Model file for the job. Use its own axes, mm. Coordinates: 2 decimals unless noted, no trailing zeros. Loops run counter-clockwise (first coordinate to the right, second up) from the corner with the lowest first, then second, coordinate; pieces in that order, holes last. Notation, with made-up numbers: (13.5, 22.25) -> (39.5, 22.25) arc R19 ccw to (39.5, 41.25) -> close; hole circle Ø11 at (40.5, -4.75). An arc over 180 degrees is marked (long way). Use one line per item in the form item = value.
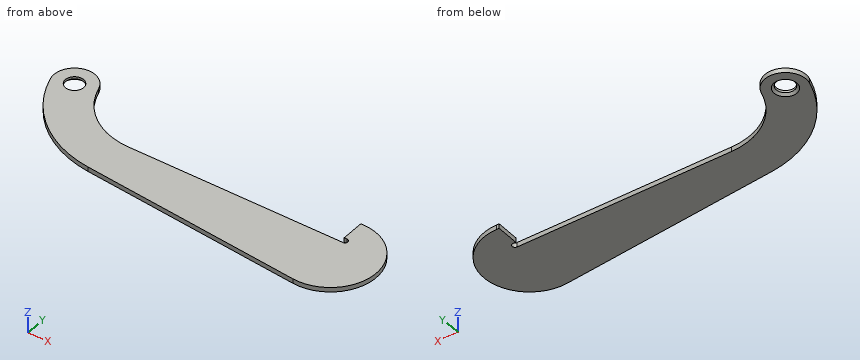
```python
from build123d import *

# Parameters (mm, degrees)
SKETCH_1_R             = 8
SM_BASE_FLANGE_1_DEPTH = 4
CHAMFER_2_SIZE         = 2


# Sheet-metal steps are written as plain solids
with BuildPart() as part:
    # Sketch 1 → Базовая кромка1 (new body)
    with BuildSketch(Plane.XY):
        with BuildLine():
            Line((259.153254995, -11.814954576), (261.653254995, -11.814954576))
            ThreePointArc((261.653254995, -11.814954576), (301.603884083, -53.801719646), (257.684629276, -91.617592804))
            Line((257.684629276, -91.617592804), (64.398882219, -72.345533941))
            ThreePointArc((64.398882219, -72.345533941), (13.404361157, -51.155129463), (-17.229741187, -5.209224379))
            ThreePointArc((-17.229741187, -5.209224379), (-5.209224379, 17.229741187), (17.229741187, 5.209224379))
            ThreePointArc((17.229741187, 5.209224379), (38.587121714, -25.160558799), (73.838171235, -36.814954576))
            Line((73.838171235, -36.814954576), (261.653254995, -36.814954576))
            ThreePointArc((261.653254995, -36.814954576), (264.153254995, -34.314954576), (261.653254995, -31.814954576))
            Line((261.653254995, -31.814954576), (259.153254995, -31.814954576))
            Line((259.153254995, -31.814954576), (259.153254995, -11.814954576))
        make_face()
        Circle(SKETCH_1_R, mode=Mode.SUBTRACT)
    extrude(amount=SM_BASE_FLANGE_1_DEPTH)

    # Фаска2
    chamfer_2_edges = [part.edges().sort_by_distance(p)[0] for p in [
        (-8, 0, 0),
    ]]
    chamfer(chamfer_2_edges, length=CHAMFER_2_SIZE)


solid = part.part
```
Q1. Pin check, flat tips, straight feed: pin 1 Ø0.8 at (x, z) = (261, 2.5) entering from +Y; pin 2 Ø1.2 at (x, z) = (260, 2.5) entering from -Y; pin 3 Ø2 at (y, z) = (-21.5, 2) entering from -X. Stop position of each tip, or through.
Result:
pin_1 = -11.81
pin_2 = -91.8
pin_3 = -11.12
Q2. Wall check: line 1 along X through (y, z) = (0, 0.2); line 2 along X through (y, z) = (-31, 3.75); line 3 along Y through (x, z) = (-5, 1.35). Give the ranges that are in metal, low to high.
Result:
line_1 = -18 to -9.8, 9.8 to 19.07
line_2 = -4.95 to 48.27, 259.15 to 295.81
line_3 = -30.93 to -7.06, 7.06 to 17.29
Q3. Band-saw the part on C-C, the plane x = 0. Write the cut outline in (y, z).
Result:
outline = (-37.67, 0) -> (-10, 0) -> (-8, 2) -> (-8, 4) -> (-37.67, 4) -> close; (8, 2) -> (10, 0) -> (18, 0) -> (18, 4) -> (8, 4) -> close
Q4. Band-saw the part on A-A, the plane y = -20. Write the cut outline in (x, z).
Result:
outline = (-11.37, 0) -> (32.53, 0) -> (32.53, 4) -> (-11.37, 4) -> close; (259.15, 0) -> (285.9, 0) -> (285.9, 4) -> (259.15, 4) -> close
Q5. Band-saw the part on B-B, the plane z = 3.1. Write the cut outline in (x, y).
Result:
outline = (-17.23, -5.21) arc R95.14 ccw to (64.4, -72.35) -> (257.68, -91.62) arc R40 ccw (long way) to (261.65, -11.81) -> (259.15, -11.81) -> (259.15, -31.81) -> (261.65, -31.81) arc R2.5 cw to (261.65, -36.81) -> (73.84, -36.81) arc R59.14 cw to (17.23, 5.21) arc R18 ccw to start; hole circle Ø16 at (0, 0)
Q6. Band-saw the part on D-D, the plane y = 0. Write the cut outline in (x, z).
Result:
outline = (-18, 0) -> (-10, 0) -> (-8, 2) -> (-8, 4) -> (-18, 4) -> close; (8, 2) -> (10, 0) -> (19.07, 0) -> (19.07, 4) -> (8, 4) -> close
